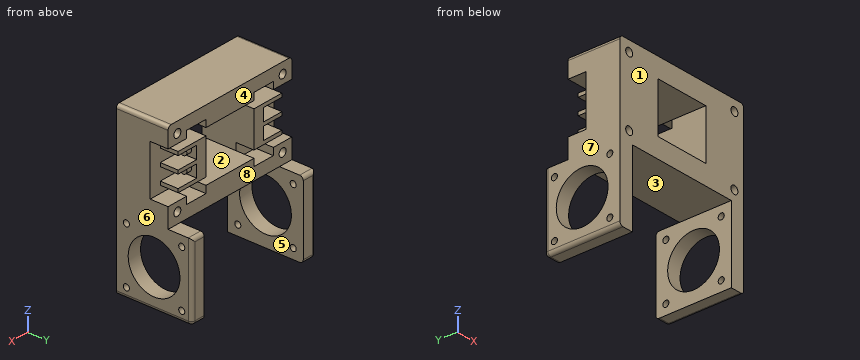
from build123d import *

# Parameters (mm, degrees)
SKETCH2_W            = 40
SKETCH2_H            = 50
BOSS_EXTRUDE1_DEPTH  = 29
CUT_EXTRUDE2_DEPTH   = 10
SKETCH6_R            = 2.085
BOSS_EXTRUDE2_DEPTH  = 3
CUT_EXTRUDE3_DEPTH   = 44.197222133
M4_CLEARANCE_HOLE2_D = 4.5
SKETCH2_3_W          = 8
SKETCH2_3_H          = 42.3
BOSS_EXTRUDE3_DEPTH  = 42.3
CUT_EXTRUDE4_REACH   = 90.986
SKETCH15_R           = 14.5
M3_CLEARANCE_HOLE1_D = 3.4
FILLET1_R            = 2
FILLET1_OF_MIRROR1_R = 2


with BuildPart() as part:
    # Sketch2 → Boss-Extrude1 (new body)
    with BuildSketch(Plane(origin=(0, 0, 0), x_dir=(1, 0, 0), z_dir=(0, 1, 0))):
        Rectangle(SKETCH2_W, SKETCH2_H)
    boss_extrude1 = extrude(amount=BOSS_EXTRUDE1_DEPTH)

    # Sketch3 → Cut-Extrude2 (cut)
    with BuildSketch(Plane(origin=(0, 29, 0), x_dir=(1, 0, 0), z_dir=(0, 1, 0))):
        Polygon((-8, 14), (-20, 14), (-20, -14), (-8, -14), (-8, -18), (4.5, -18), (4.5, -14), (4.5, -10), (-13.5, -10), (-13.5, -8), (-1.5, -8), (-1.5, -1), (-13.5, -1), (-13.5, 1), (-1.5, 1), (-1.5, 8), (-13.5, 8), (-13.5, 10), (4.5, 10), (4.5, 14), (4.5, 18), (-8, 18), align=None)
    cut_extrude2 = extrude(amount=-CUT_EXTRUDE2_DEPTH, mode=Mode.SUBTRACT)

    # Sketch6 → Boss-Extrude2 (add)
    with BuildSketch(Plane.ZY.offset(1.5)):
        with Locations((-4.5, 24)):
            Circle(SKETCH6_R)
        with Locations((4.5, 24)):
            Circle(SKETCH6_R)
    boss_extrude2 = extrude(amount=BOSS_EXTRUDE2_DEPTH)

    # Sketch3<4> → Cut-Extrude3 (cut, through all)
    with BuildSketch(Plane(origin=(0, 29, 0), x_dir=(1, 0, 0), z_dir=(0, 1, 0))):
        Polygon((20, -14), (20, 14), (4.5, 14), (4.5, 10), (4.5, -10), (4.5, -14), align=None)
    cut_extrude3 = extrude(amount=-CUT_EXTRUDE3_DEPTH, mode=Mode.SUBTRACT)

    # M4 Clearance Hole2 (through all)
    with Locations(Plane(origin=(0, 29, 0), x_dir=(1, 0, 0), z_dir=(0, 1, 0))):
        with Locations((-14, -19), (-14, 19)):
            m4_clearance_hole2 = Hole(M4_CLEARANCE_HOLE2_D / 2)

    # Sketch2<3> → Boss-Extrude3 (add)
    with BuildSketch(Plane(origin=(0, 0, 0), x_dir=(1, 0, 0), z_dir=(0, 1, 0))):
        with Locations((-16, 46.15)):
            Rectangle(SKETCH2_3_W, SKETCH2_3_H)
    boss_extrude3 = extrude(amount=BOSS_EXTRUDE3_DEPTH)

    # Sketch15 → Cut-Extrude4 (cut, up to next)
    with BuildSketch(Plane.ZY.offset(20), mode=Mode.PRIVATE) as cut_extrude4_sk1:
        with Locations((-46.15, 21.15)):
            Circle(SKETCH15_R)
    cut_extrude4_tool1 = extrude(cut_extrude4_sk1.sketch, amount=-CUT_EXTRUDE4_REACH, mode=Mode.PRIVATE) & part.part
    cut_extrude4 = cut_extrude4_tool1.solids().sort_by_distance((-20, 21.15, -46.15))[0]
    add(cut_extrude4, mode=Mode.SUBTRACT)

    # M3 Clearance Hole1 (through all)
    with Locations(Plane(origin=(-12, 0, 0), x_dir=(0, 0, 1), z_dir=(1, 0, 0))):
        with Locations((-61.65, -36.65), (-30.65, -36.65), (-61.65, -5.65), (-30.65, -5.65)):
            m3_clearance_hole1 = Hole(M3_CLEARANCE_HOLE1_D / 2)

    # Fillet1
    fillet1_edges = [part.edges().sort_by_distance(p)[0] for p in [
        (-16, 42.3, -67.3),
        (-20, 42.3, -46.15),
        (-20, 21.15, -67.3),
        (-16, 42.3, -25),
        (-20, 14.5, 25),
    ]]
    fillet(fillet1_edges, radius=FILLET1_R)

    # Mirror1: Boss-Extrude1, Cut-Extrude2, Boss-Extrude2, Cut-Extrude3, M4 Clearance Hole2, Boss-Extrude3, Cut-Extrude4, M3 Clearance Hole1 across plane
    add(boss_extrude1.mirror(Plane(origin=(20, 0, 0), x_dir=(0, 0, 1), z_dir=(1, 0, 0))))
    add(cut_extrude2.mirror(Plane(origin=(20, 0, 0), x_dir=(0, 0, 1), z_dir=(1, 0, 0))), mode=Mode.SUBTRACT)
    add(boss_extrude2.mirror(Plane(origin=(20, 0, 0), x_dir=(0, 0, 1), z_dir=(1, 0, 0))))
    add(cut_extrude3.mirror(Plane(origin=(20, 0, 0), x_dir=(0, 0, 1), z_dir=(1, 0, 0))), mode=Mode.SUBTRACT)
    add(m4_clearance_hole2.mirror(Plane(origin=(20, 0, 0), x_dir=(0, 0, 1), z_dir=(1, 0, 0))), mode=Mode.SUBTRACT)
    add(boss_extrude3.mirror(Plane(origin=(20, 0, 0), x_dir=(0, 0, 1), z_dir=(1, 0, 0))))
    add(cut_extrude4.mirror(Plane(origin=(20, 0, 0), x_dir=(0, 0, 1), z_dir=(1, 0, 0))), mode=Mode.SUBTRACT)
    add(m3_clearance_hole1.mirror(Plane(origin=(20, 0, 0), x_dir=(0, 0, 1), z_dir=(1, 0, 0))), mode=Mode.SUBTRACT)

    # Fillet1 of Mirror1
    fillet1_of_mirror1_edges = [part.edges().sort_by_distance(p)[0] for p in [
        (56, 42.3, -67.3),
        (60, 42.3, -46.15),
        (60, 21.15, -67.3),
        (56, 42.3, -25),
        (60, 14.5, 25),
    ]]
    fillet(fillet1_of_mirror1_edges, radius=FILLET1_OF_MIRROR1_R)


solid = part.part
Build history of the part. All positions in model axes, mm. Face numbers are marked on the shaded views. A direction names the side the tool comes from. Coordinates: 2 decimals unless noted, no trailing zeros. Write each loop counter-clockwise with the first axis right and the second up, starting at its lowest first coordinate (ties: lowest second). Pieces come first, ordered by that corner, then holes.
(1) Cut at B-B on z = -46.15. List the corners of the cut face in (x, y), and give its area (3 significant figures).
(2) Cut at D-D on y = 27.5. State how many separate pieces and enclosed holes the cut face has, and give its area (3 significant figures).
(3) Mould opens along X. For the marked faces 5, 6, 7 and 8 say: pulls with the +X half, pulls with the -X half, needs draft (parallel to the pull), parting line crosses it, or undercut.
(4) Drill centre lines: line 1 (Y direction, x = 57, z = -61.65); line 2 (X direction, y = 28, z = -15.5); line 3 (Z direction, x = 55, y = 6). Where is each one in solid material? Low to high.
(5) Cut at A-A on x = 19.5. List the corners of the cut face in (y, z), and give its area (3 significant figures).
(6) 3-axis set-ups, long thin cutter, end or side, ignore diameter. For the marked faces 1, 2, 3 and 4: which of +Z, -Z, +X, -X, +Y, -Y reach the whole face in a straight line?
(7) Pin check, flat tips, straight feed: pin 1 Ø0.6 at (y, z) = (25, 8.5) entering from -X; pin 2 Ø1 at (x, y) = (20, 14) entering from -Z; pin 3 Ø12 at (x, z) = (36.5, -20.5) entering from +Y. Stop position of each tip, or through.
(8) Cut at C-C on z = 4.5. List the corners of the cut face in (x, y) (3 decimals).
Working result:
1. outline: (-20, 0) - (-12, 0) - (-12, 6.65) - (-20, 6.65) - close; (-20, 35.65) - (-12, 35.65) - (-12, 42.3) - (-18, 42.3) arc R2 ccw to (-20, 40.3) - close; (52, 0) - (60, 0) - (60, 6.65) - (52, 6.65) - close; (52, 35.65) - (60, 35.65) - (60, 40.3) arc R2 ccw to (58, 42.3) - (52, 42.3) - close
1. area: 211 mm2
2. separate pieces: 6
2. enclosed holes: 4
2. area: 2,140 mm2
3. face 5: undercut
3. face 6: pulls with the +X half
3. face 7: pulls with the -X half
3. face 8: needs draft
4. line 1: y = 0 to 3.95, 7.35 to 34.95, 38.35 to 42.3
4. line 2: x = -20 to -8, 4.5 to 35.5, 48 to 60
4. line 3: z = -67.3 to -63.31, -59.99 to -32.31, -28.99 to -21.02, -16.98 to 16.98, 21.02 to 25
5. outline: (0, -25) - (29, -25) - (29, -14) - (0, -14) - close; (0, 14) - (29, 14) - (29, 25) - (0, 25) - close
5. area: 638 mm2
6. face 1: +Z, -Z, +X, -X, -Y
6. face 2: +Y, -Y
6. face 3: -Z, +Y, -Y
6. face 4: +Z, +X, -X, +Y
7. pin 1: stops at x = -13.5
7. pin 2: stops at z = -25
7. pin 3: stops at y = 29
8. outline: (-20, 0) - (4.5, 0) - (4.5, 29) - (-1.5, 29) - (-1.5, 26.085) - (-4.5, 26.085) - (-4.5, 21.915) - (-1.5, 21.915) - (-1.5, 19) - (-20, 19) - close; (35.5, 0) - (60, 0) - (60, 19) - (41.5, 19) - (41.5, 21.915) - (44.5, 21.915) - (44.5, 26.085) - (41.5, 26.085) - (41.5, 29) - (35.5, 29) - close
